from build123d import *

# Parameters (mm, degrees)
SKETCH1_W           = 30
SKETCH1_H           = 30
EXTRUDE1_DEPTH      = 2.5
FILLET2_R           = 3
SKETCH3_R           = 10.2
SKETCH3_R_2         = 9.4
EXTRUDE2_DEPTH      = 11.3
EXTRUDE3_DEPTH      = 4.9
EXTRUDE3_DEPTH_BACK = 6.7
SKETCH4_R           = 8
EXTRUDE4_DEPTH      = 5.9
EXTRUDE4_DEPTH_BACK = 17
SKETCH5_R           = 0.9
FILLET3_R           = 0.9
SKETCH6_R           = 10.05
SKETCH6_R_2         = 9.55
EXTRUDE5_DEPTH      = 6.7
CUT_EXTRUDE1_DEPTH  = 5
SKETCH8_R           = 9.55
SKETCH8_R_2         = 8
EXTRUDE7_DEPTH      = 5.5
CUT_EXTRUDE2_DEPTH  = 1


with BuildPart() as part:
    # Sketch1 → Extrude1 (new body)
    with BuildSketch(Plane(origin=(0, 0, 0), x_dir=(1, 0, 0), z_dir=(0, 1, 0))):
        Rectangle(SKETCH1_W, SKETCH1_H)
        with BuildLine():
            Line((13.409009742, 11.641242789), (10.580582618, 8.812815665))
            ThreePointArc((10.580582618, 8.812815665), (8.812815665, 8.812815665), (8.812815665, 10.580582618))
            Line((8.812815665, 10.580582618), (11.641242789, 13.409009742))
            ThreePointArc((11.641242789, 13.409009742), (13.409009742, 13.409009742), (13.409009742, 11.641242789))
        make_face(mode=Mode.SUBTRACT)
        with BuildLine():
            Line((-13.409009742, 11.641242789), (-10.580582618, 8.812815665))
            ThreePointArc((-10.580582618, 8.812815665), (-8.812815665, 8.812815665), (-8.812815665, 10.580582618))
            Line((-8.812815665, 10.580582618), (-11.641242789, 13.409009742))
            ThreePointArc((-11.641242789, 13.409009742), (-13.409009742, 13.409009742), (-13.409009742, 11.641242789))
        make_face(mode=Mode.SUBTRACT)
        with BuildLine():
            Line((-11.641242789, -13.409009742), (-8.812815665, -10.580582618))
            ThreePointArc((-8.812815665, -10.580582618), (-8.812815665, -8.812815665), (-10.580582618, -8.812815665))
            Line((-10.580582618, -8.812815665), (-13.409009742, -11.641242789))
            ThreePointArc((-13.409009742, -11.641242789), (-13.409009742, -13.409009742), (-11.641242789, -13.409009742))
        make_face(mode=Mode.SUBTRACT)
        with BuildLine():
            Line((11.641242789, -13.409009742), (8.812815665, -10.580582618))
            ThreePointArc((8.812815665, -10.580582618), (8.812815665, -8.812815665), (10.580582618, -8.812815665))
            Line((10.580582618, -8.812815665), (13.409009742, -11.641242789))
            ThreePointArc((13.409009742, -11.641242789), (13.409009742, -13.409009742), (11.641242789, -13.409009742))
        make_face(mode=Mode.SUBTRACT)
    extrude(amount=EXTRUDE1_DEPTH)

    # Fillet2
    fillet2_edges = [part.edges().sort_by_distance(p)[0] for p in [
        (15, 1.25, 15),
        (-15, 1.25, 15),
        (-15, 1.25, -15),
        (15, 1.25, -15),
    ]]
    fillet(fillet2_edges, radius=FILLET2_R)

    # Sketch3 → Extrude2 (add)
    with BuildSketch(Plane(origin=(0, 2.5, 0), x_dir=(1, 0, 0), z_dir=(0, 1, 0))):
        with Locations(Location((0, 0, 0), (0, 0, 270))):
            Circle(SKETCH3_R)
        with Locations(Location((0, 0, 0), (0, 0, 270))):
            Circle(SKETCH3_R_2, mode=Mode.SUBTRACT)
    extrude(amount=EXTRUDE2_DEPTH)

    # Sketch4 → Extrude3 (add, two sides: drawn at the far end of the back side and taken through both)
    with BuildSketch(Plane(origin=(0, 2.5, 0), x_dir=(1, 0, 0), z_dir=(0, 1, 0)).offset(-EXTRUDE3_DEPTH_BACK)):
        with Locations(Location((0, 0, 0), (0, 0, 270))):
            Circle(SKETCH4_R)
    extrude(amount=EXTRUDE3_DEPTH + EXTRUDE3_DEPTH_BACK)

    # Sketch5 → Extrude4 (add, two sides: drawn at the far end of the back side and taken through both)
    with BuildSketch(Plane(origin=(0, 7.4, 0), x_dir=(1, 0, 0), z_dir=(0, 1, 0)).offset(-EXTRUDE4_DEPTH_BACK)):
        with Locations(Location((3.4, 0, 0), (0, 0, 270))):
            Circle(SKETCH5_R)
        with Locations(Location((-3.4, 0, 0), (0, 0, 270))):
            Circle(SKETCH5_R)
    extrude(amount=EXTRUDE4_DEPTH + EXTRUDE4_DEPTH_BACK)

    # Fillet3
    fillet3_edges = [part.edges().sort_by_distance(p)[0] for p in [
        (3.4, 13.3, -0.9),
        (-3.4, 13.3, -0.9),
    ]]
    fillet(fillet3_edges, radius=FILLET3_R)

    # Sketch6 → Extrude5 (add)
    with BuildSketch(Plane.XZ):
        with Locations(Location((0, 0, 0), (0, 0, 90))):
            Circle(SKETCH6_R)
        with Locations(Location((0, 0, 0), (0, 0, 270))):
            Circle(SKETCH6_R_2, mode=Mode.SUBTRACT)
    extrude(amount=EXTRUDE5_DEPTH)

    # Sketch7 → Cut-Extrude1 (cut)
    with BuildSketch(Plane.XZ.offset(9.6)):
        with BuildLine():
            Line((3.4, 0.9), (3.4, 0.6))
            ThreePointArc((3.4, 0.6), (2.8, 0), (3.4, -0.6))
            Line((3.4, -0.6), (3.4, -0.9))
            ThreePointArc((3.4, -0.9), (4.3, 0), (3.4, 0.9))
        make_face()
        with BuildLine():
            Line((-3.4, -0.6), (-3.4, -0.9))
            ThreePointArc((-3.4, -0.9), (-2.5, 0), (-3.4, 0.9))
            Line((-3.4, 0.9), (-3.4, 0.6))
            ThreePointArc((-3.4, 0.6), (-4, 0), (-3.4, -0.6))
        make_face()
    extrude(amount=-CUT_EXTRUDE1_DEPTH, mode=Mode.SUBTRACT)

    # Sketch8 → Extrude7 (add)
    with BuildSketch(Plane.XZ):
        with Locations(Location((0, 0, 0), (0, 0, 270))):
            Circle(SKETCH8_R)
        with Locations(Location((0, 0, 0), (0, 0, 90))):
            Circle(SKETCH8_R_2, mode=Mode.SUBTRACT)
    extrude(amount=EXTRUDE7_DEPTH)

    # Sketch9 → Cut-Extrude2 (cut)
    with BuildSketch(Plane.XZ.offset(5.5)):
        Polygon((-4.635007145, -8.409471372), (6.276512407, 7.26690388), (4.635007145, 8.409471372), (-6.276512407, -7.26690388), align=None)
    extrude(amount=-CUT_EXTRUDE2_DEPTH, mode=Mode.SUBTRACT)


solid = part.part
Design review of the part built by this model. Coordinates are the model's own, in mm. A direction names the side the tool comes from. Round coordinates to 2 decimals unless told otherwise and drop trailing zeros. Loops run counter-clockwise (first coordinate to the right, second up) from the corner with the lowest first, then second, coordinate; pieces in that order, holes last. Notation, with made-up numbers: (5, 29.25) - (19, 29.25) arc R26 ccw to (19, 45.25) - close; hole circle Ø1 at (-16.5, 35.5). An arc over 180 degrees is marked (long way). One line per item, written item: value. Start each with the question number.
1) Draft analysis for pull direction Z (two halves, no side actions). For faces 1 (the flat face through (5, -4.5, 7)), 2 (the cylindrical face through (-14.14, 1.27, -14.1)), 3 (the flat face through (-7, 13.8, 7)), state which applies: +Z half, -Z half, draft (parallel to the pull), parting line (faces both ways), or undercut.
2) Consider section D-D on y = 3. Give the boundary of the cut face in (x, z), then the cut area to 3 significant figures.
3) Consider section B-B on z = 13. Give the boundary of the cut face in (x, y), then the cut area to 3 significant figures.
4) Consider section A-A on y = -7.5. Give the boundary of the cut face in (x, z), then the cut area to 3 significant figures.
5) For faces 4 (the cylindrical face through (2.521, 9.865, -0.195)), 5 (the cylindrical face through (7.81, -4.84, -1.73)), 6 (the flat face through (5.47, -5.01, 7.83)), 7 (the flat face through (-11.975, 1.232, 10.207)), 8 (the flat face through (-15, 1, 0)), list the 3-axis set-ups (+Z, -Z, +X, -X, +Y, -Y) from which the entire face can be reached by the end or side of a thin tool; tool diameter is ignored.
6) Consider section C-C on x = -13. Give the boundary of the cut face in (y, z), then the cut area to 3 significant figures.
7) To check wall thickness, follow L1, parallel to X at y = -6, z = 0; L2, parallel to X at y = -5, z = 0; L3, parallel to X at y = 5.75, z = 2.5. State the ranges of each line that lie inside material, in increasing order. Write a range as from..to.
8) Insertion check: pin 1 Ø2.5 at (x, z) = (-5, -7) entering from -Y; pin 2 Ø2 at (x, z) = (-2, 1) entering from +Y; pin 3 Ø5.5 at (x, z) = (-3.5, 1) entering from +Y. Each pin has a flat end and moves straight along its axis. Give the tip position at first contact, or say it passes through.
Reported:
1. face 1: undercut
1. face 2: -Z half
1. face 3: draft
2. outline: circle Ø20.4 at (0, 0); circle Ø16 at (0, 0); hole circle Ø18.8 at (0, 0)
2. area: 250 mm^2
3. outline: (-14.83, 0) - (-13.68, 0) - (-13.68, 2.5) - (-14.83, 2.5) - close; (-11.23, 0) - (11.23, 0) - (11.23, 2.5) - (-11.23, 2.5) - close; (13.68, 0) - (14.83, 0) - (14.83, 2.5) - (13.68, 2.5) - close
3. area: 61.9 mm^2
4. outline: (-3.4, -0.9) - (-3.4, -0.6) arc R0.6 cw to (-3.4, 0.6) - (-3.4, 0.9) arc R0.9 ccw to start; (3.4, -0.9) - (3.4, -0.6) arc R0.6 cw to (3.4, 0.6) - (3.4, 0.9) arc R0.9 ccw to start
4. area: 1.41 mm^2
5. face 4: +Y
5. face 5: -Y
5. face 6: none
5. face 7: +Y, -Y
5. face 8: +Z, -Z, -X, +Y, -Y
6. outline: (0, -14.83) - (2.5, -14.83) - (2.5, -13.68) - (0, -13.68) - close; (0, -11.23) - (2.5, -11.23) - (2.5, 11.23) - (0, 11.23) - close; (0, 13.68) - (2.5, 13.68) - (2.5, 14.83) - (0, 14.83) - close
6. area: 61.9 mm^2
7. L1: x = -10.05..-9.55, -4.3..-4, 2.5..2.8, 9.55..10.05
7. L2: x = -10.05..-8, -4.3..-4, 2.5..2.8, 8..10.05
7. L3: x = -9.89..-9.06, -7.6..7.6, 9.06..9.89
8. pin 1: stops at y = -6.7
8. pin 2: stops at y = 12.94
8. pin 3: stops at y = 13.3
